The listing builds one solid part. Answer for the finished solid, in the listing's coordinates (mm). A direction names the side the tool comes from. Round coordinates to 2 decimals unless told otherwise and drop trailing zeros. Write each loop counter-clockwise with the first axis right and the second up, starting at its lowest first coordinate (ties: lowest second). Pieces come first, ordered by that corner, then holes. Notation, with made-up numbers: (-33, -10) - (-17, -10) arc R8 ccw to (-17, -6) - close; hole circle Ø8 at (-2, 58.5). An arc over 180 degrees is marked (long way). Return JSON: item names as keys, results as strings. Group by question number.
(1) Section D-D, the plane x = 3 is taken. Write down the section's boundary in (y, z), then the cut area to 3 significant figures.
(2) Determine the mould class of faces 1 (the flat face through (7.642, 14.79, 1.521)), 2 (the cylindrical face through (-0.38, 12.56, -10.34)), 3 (the flat face through (0.5, 0, -5.5)), 4 (the flat face through (0.5, 30, -5.5)) for opening direction Y: +Y half, -Y half, draft (parallel to the pull), parting line (faces both ways), or undercut.
(3) Find the intervals of material crossed by line 1 along Z through (x, y) = (-1.15, 15); line 2 along Y through (x, z) = (-1.2, -9.8); line 3 along X through (y, z) = (17, -14), in increasing order. Write a range as [from, to].
(4) Section A-A, the plane z = -9.8 is taken. Write down the section's boundary in (x, y), then the cut area to 3 significant figures.
(5) Section B-B, the plane y = 15 is taken. Write down the section's boundary in (x, z), then the cut area to 3 significant figures.
(6) Section C-C, the plane y = 8.5 is taken. Write down the section's boundary in (x, z), then the cut area to 3 significant figures.
(7) Which of the six approach directions +Z, -Z, +X, -X, +Y, -Y give full straight-line access (tool end or side, diameter ignored) to faces 5 (the flat face through (5, 15, 0)), 6 (the flat face through (0, 15, -1)), 7 (the flat face through (4, 15, 3))?
(8) Each of these flat-tipped pins is pushed along its axis until it touches: pin 1 (3 mm diameter, centred on y = 5, z = -13, fed in from +X); pin 2 (6 mm diameter, centred on x = 2, y = 24, fed in from -Z); pin 3 (0.5 mm diameter, centred on y = 20, z = -1, fed in from -X); pin 4 (3.5 mm diameter, centred on x = 4, y = 17, fed in from -Z). Where does it stop, or does it pass through?
```python
from build123d import *

# Parameters (mm, degrees)
EXTRUDE_1_DEPTH          = 30
CUT_EXTRUDE_1_DEPTH      = 36.836433974
CUT_EXTRUDE_1_DEPTH_BACK = 36.836433974
SKETCH_2_R               = 2.5


with BuildPart() as part:
    # 草图1 → 凸台-拉伸1 (new body)
    with BuildSketch(Plane(origin=(0, 0, 0), x_dir=(1, 0, 0), z_dir=(0, 1, 0))):
        Polygon((0, 1.8), (0, 0), (1.1, 0), (1.1, 16.8), (-1.9, 16.8), (-1.9, 1.8), align=None)
        Polygon((1.1, -3), (7.1, -3), (8.2, 0), (0, 0), align=None)
    extrude(amount=EXTRUDE_1_DEPTH)

    # 草图2 → 切除-拉伸1 (cut, two sides: drawn at the far end of the back side and taken through both)
    with BuildSketch(Plane.ZY.offset(1.9).offset(-CUT_EXTRUDE_1_DEPTH_BACK)):
        with Locations((-9.8, 15)):
            Circle(SKETCH_2_R)
    extrude(amount=CUT_EXTRUDE_1_DEPTH + CUT_EXTRUDE_1_DEPTH_BACK, mode=Mode.SUBTRACT)


solid = part.part
```
Working result:
{
 "1": {"outline": "(0, 0) - (30, 0) - (30, 3) - (0, 3) - close", "area": "90.0 mm^2"},
 "2": {"face 1": "draft", "face 2": "undercut", "face 3": "-Y half", "face 4": "+Y half"},
 "3": {"line 1": "z = [-16.8, -12.3], [-7.3, -1.8]", "line 2": "y = [0, 12.5], [17.5, 30]", "line 3": "x = [-1.9, 1.1]"},
 "4": {"outline": "(-1.9, 0) - (1.1, 0) - (1.1, 12.5) - (-1.9, 12.5) - close; (-1.9, 17.5) - (1.1, 17.5) - (1.1, 30) - (-1.9, 30) - close", "area": "75.0 mm^2"},
 "5": {"outline": "(-1.9, -16.8) - (1.1, -16.8) - (1.1, -12.3) - (-1.9, -12.3) - close; (-1.9, -7.3) - (1.1, -7.3) - (1.1, 0) - (8.2, 0) - (7.1, 3) - (1.1, 3) - (0, 0) - (0, -1.8) - (-1.9, -1.8) - close", "area": "53.3 mm^2"},
 "6": {"outline": "(-1.9, -16.8) - (1.1, -16.8) - (1.1, 0) - (8.2, 0) - (7.1, 3) - (1.1, 3) - (0, 0) - (0, -1.8) - (-1.9, -1.8) - close", "area": "68.3 mm^2"},
 "7": {"face 5": "-Z, +X, +Y, -Y", "face 6": "+Z, -X, +Y, -Y", "face 7": "+Z, +X, -X, +Y, -Y"},
 "8": {"pin 1": "stops at x = 1.1", "pin 2": "stops at z = -16.8", "pin 3": "stops at x = 0", "pin 4": "stops at z = 0"}
}
